Job drawing, mm, ordinate dimensions from the low corner. One solid piece. Round coordinates to 2 decimals unless told otherwise and drop trailing zeros. Order: outer loops, then holes, each group sorted by start corner. A loop starts at its lowest first (then second) coordinate and runs counter-clockwise, first axis right, second up. Notation, with made-up numbers: (29.5, 88) -> (33.5, 88) arc R8 cw to (33.5, 99) -> close; hole circle Ø11 at (68.5, 86.25). An arc over 180 degrees is marked (long way). Answer as a JSON object with one key per item and string values. Group by question number.
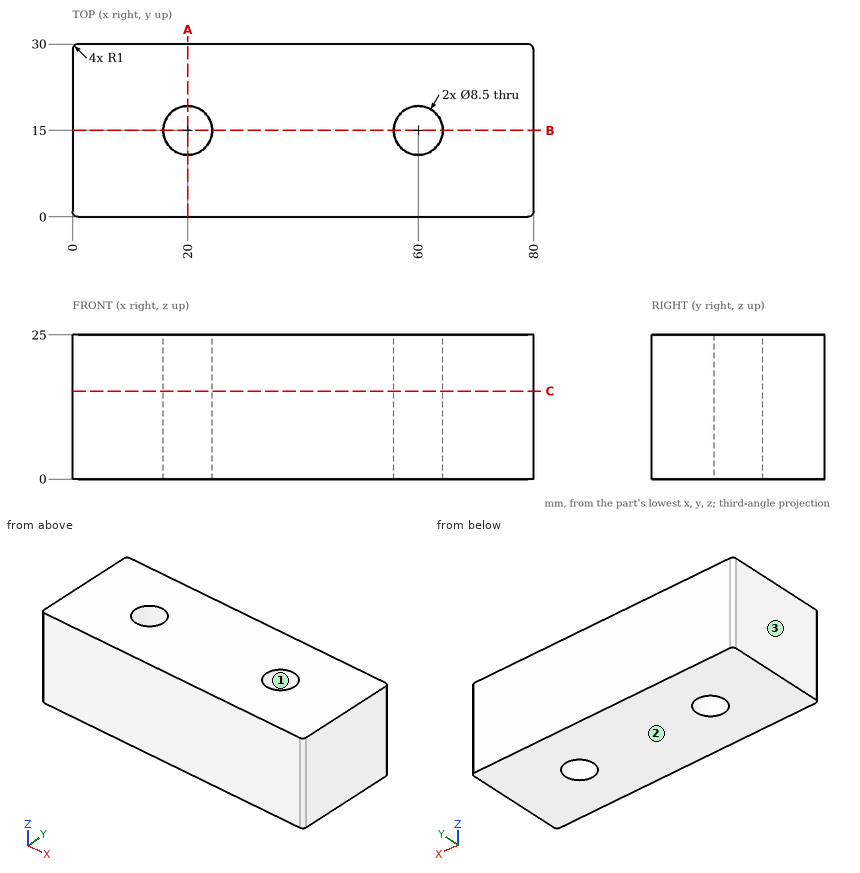
Q1. Two-plate mould, pull along X, no slides. Class the marked faces 1, 2 and 3: +X half, -X half, draft (parallel to the pull), parting line (faces both ways), or undercut.
Q2. Band-saw the part on B-B (y = 15). List the corners of the cut face in (x, z).
Q3. Drop a flat-ended pin along its axis: pin 1 Ø7 at (x, y) = (60, 15) entering from +Z. Give the stop position or say it passes through.
Q4. Wall check: line 1 (X direction, y = 15, z = 10.5); line 2 (X direction, y = 18.75, z = 1.5); line 3 (Y direction, x = 60, z = 5). Give the ranges that are in metal, low to high. Write a range as [from, to].
Q5. Band-saw the part on A-A (x = 20). List the corners of the cut face in (y, z), plus the area to 4 significant figures.
Q6. Band-saw the part on C-C (z = 15.25). List the corners of the cut face in (x, y), plus the area to 3 significant figures.
Completed:
{
 "1": {"face 1": "undercut", "face 2": "draft", "face 3": "-X half"},
 "2": {"outline": "(0, 0) -> (15.75, 0) -> (15.75, 25) -> (0, 25) -> close; (24.25, 0) -> (55.75, 0) -> (55.75, 25) -> (24.25, 25) -> close; (64.25, 0) -> (80, 0) -> (80, 25) -> (64.25, 25) -> close"},
 "3": {"pin 1": "through"},
 "4": {"line 1": "[0, 15.75], [24.25, 55.75], [64.25, 80]", "line 2": "[0, 18], [22, 58], [62, 80]", "line 3": "[0, 10.75], [19.25, 30]"},
 "5": {"outline": "(0, 0) -> (10.75, 0) -> (10.75, 25) -> (0, 25) -> close; (19.25, 0) -> (30, 0) -> (30, 25) -> (19.25, 25) -> close", "area": "537.5 mm2"},
 "6": {"outline": "(0, 1) arc R1 ccw to (1, 0) -> (79, 0) arc R1 ccw to (80, 1) -> (80, 29) arc R1 ccw to (79, 30) -> (1, 30) arc R1 ccw to (0, 29) -> close; hole circle Ø8.5 at (20, 15); hole circle Ø8.5 at (60, 15)", "area": "2,290 mm2"}
}
